For this review, use the dimensioned drawing (mm, ordinates from the lowest corner) and the shaded views. A direction names the side the tool comes from. Coordinates: 2 decimals unless noted, no trailing zeros. Loops run counter-clockwise (first coordinate to the right, second up) from the corner with the lowest first, then second, coordinate; pieces in that order, holes last. Notation, with made-up numbers: M 56.25,12 L 98.25,12 A15 ccw 98.25,31 Z; hole C 68.25,-5 d11. An arc over 180 degrees is marked long. One line per item, written item: value.
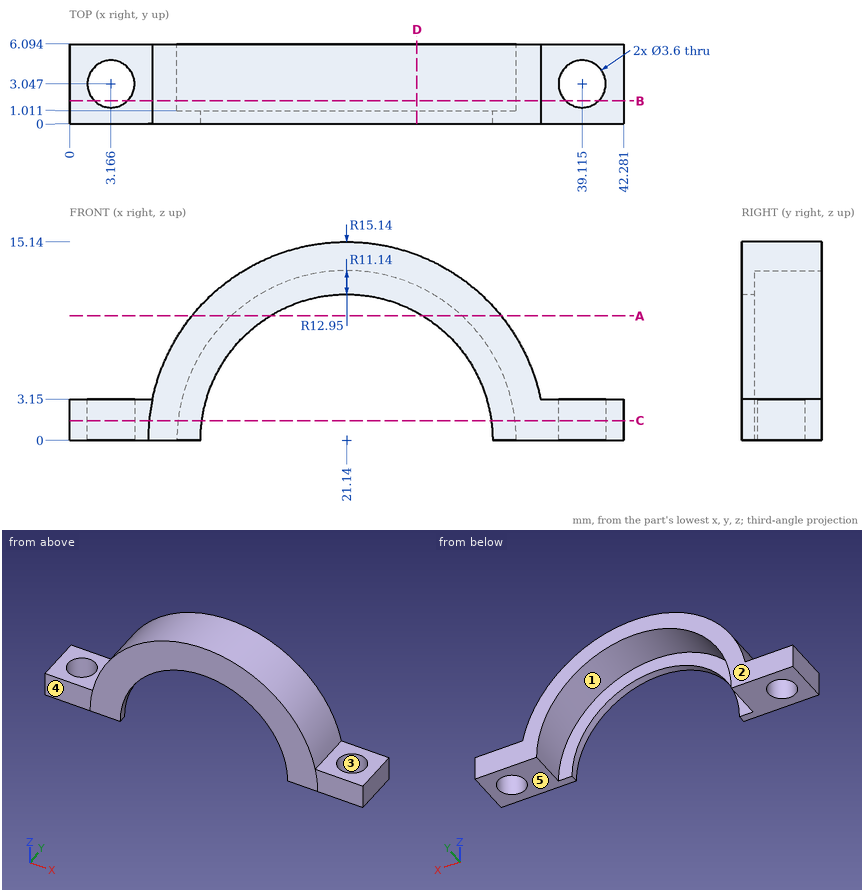
(1) Tool access review of the marked faces 1 and 2: name each direction out of +Z, -Z, +X, -X, +Y, -Y from which nothing blocks a thin tool from reaching the whole face with its end or side.
Reply:
face 1: -Z, +Y
face 2: +Z, -Z, +X, -X, +Y
(2) We need section A-A on z = 9.5. State the section outline as (x, y) points.
Reply:
outline: M 9.35,0 L 15.32,0 L 15.32,1.01 L 12.34,1.01 L 12.34,6.09 L 9.35,6.09 Z; M 26.96,0 L 32.93,0 L 32.93,6.09 L 29.94,6.09 L 29.94,1.01 L 26.96,1.01 Z
(3) We need section B-B on y = 1.75. State the section outline as (x, z) points.
Reply:
outline: M 0,0 L 1.92,0 L 1.92,3.15 L 0,3.15 Z; M 4.41,0 L 8.19,0 A12.95 cw 34.09,0 L 37.87,0 L 37.87,3.15 L 35.95,3.15 A15.14 ccw 6.33,3.15 L 4.41,3.15 Z; M 40.36,0 L 42.28,0 L 42.28,3.15 L 40.36,3.15 Z
(4) Mouldability with a two-part tool opening along Y and no side actions: class the marked faces 3, 4 and 5 as released by +Y, released by -Y, zero draft, split by the parting line, or undercut.
Reply:
face 3: undercut
face 4: released by -Y
face 5: zero draft
(5) We need section C-C on z = 1.5. State the section outline as (x, y) points (1 decimal).
Reply:
outline: M 0,0 L 10.1,0 L 10.1,1 L 8.3,1 L 8.3,6.1 L 0,6.1 Z; M 32.2,0 L 42.3,0 L 42.3,6.1 L 34,6.1 L 34,1 L 32.2,1 Z; hole C 3.2,3 d3.6; hole C 39.1,3 d3.6
(6) Insertion check: pin 1 (2 mm diameter, centred on y = 1.5, z = 4.5, fed in from -X); pin 2 (3 mm diameter, centred on x = 18, y = 4.5, fed in from +Z); pin 3 (3 mm diameter, centred on x = 35, y = 2.5, fed in from +Z) (1 decimal). Each pin has a flat end and moves straight along its axis. Give the tip position at first contact, or say it passes through.
Reply:
pin 1: stops at x = 6.41
pin 2: stops at z = 15.05
pin 3: stops at z = 8.7
(7) To check wall thickness, follow line 1 along X through (y, z) = (2, 1); line 2 along Y through (x, z) = (12.5, 7.75); line 3 along X through (y, z) = (2.75, 2) (1 decimal). State the ranges of each line that lie inside material, in increasing order. Write a range as [from, to].
Reply:
line 1: x = [0, 1.7], [4.63, 8.23], [34.05, 37.65], [40.58, 42.28]
line 2: y = [0, 1.01]
line 3: x = [0, 1.4], [4.9, 8.3], [33.9, 37.3], [40.9, 42.3]
(8) We need section D-D on x = 26.5. State the section outline as (y, z) points.
Reply:
outline: M 0,9.77 L 1.01,9.77 L 1.01,11.79 L 6.09,11.79 L 6.09,14.16 L 0,14.16 Z
